Autodesk Inventor part; units mm, degrees
ref_plane "YZ Plane" through (0, 0, 0) normal (1, 0, 0) x (0, 1, 0)
ref_plane "XZ Plane" through (0, 0, 0) normal (0, 1, 0) x (-1, 0, 0)
ref_plane "XY Plane" through (0, 0, 0) normal (0, 0, 1) x (1, 0, 0)
sketch "Sketch1" plane through (0, 0, 0) normal (0, 1, 0) x (-1, 0, 0)
  arc A0 (-2.8605, -1.9692) -> (-1.9692, -2.8605) centre (-2.4696, -2.4696) ccw
  line L0 (-1.3405, -2.2319) -> (-1.9692, -2.8605)
  arc A1 (-1.3405, -2.2319) -> (1.3405, -2.2319) centre (0, 0) ccw
  line L1 (1.9692, -2.8605) -> (1.3405, -2.2319)
  arc A2 (1.9692, -2.8605) -> (2.8605, -1.9692) centre (2.4696, -2.4696) ccw
  line L2 (2.2319, -1.3405) -> (2.8605, -1.9692)
  arc A3 (2.2319, -1.3405) -> (2.2319, 1.3405) centre (0, 0) ccw
  line L3 (2.8605, 1.9692) -> (2.2319, 1.3405)
  arc A4 (2.8605, 1.9692) -> (1.9692, 2.8605) centre (2.4696, 2.4696) ccw
  line L4 (1.3405, 2.2319) -> (1.9692, 2.8605)
  arc A5 (1.3405, 2.2319) -> (-1.3405, 2.2319) centre (0, 0) ccw
  line L5 (-1.9692, 2.8605) -> (-1.3405, 2.2319)
  arc A6 (-1.9692, 2.8605) -> (-2.8605, 1.9692) centre (-2.4696, 2.4696) ccw
  line L6 (-2.2319, 1.3405) -> (-2.8605, 1.9692)
  arc A7 (-2.2319, 1.3405) -> (-2.2319, -1.3405) centre (0, 0) ccw
  line L7 (-2.8605, -1.9692) -> (-2.2319, -1.3405)
  arc A8 (4.5171, -1.6395) -> (5.447, -3.8845) centre (7.6921, -1.6395) ccw
  line L8 (8.7557, -7.1932) -> (5.447, -3.8845)
  arc A9 (8.7557, -7.1932) -> (10.4901, -6.4748) centre (9.4741, -6.4748) ccw
  line L9 (10.4901, 6.4748) -> (10.4901, -6.4748)
  arc A10 (10.4901, 6.4748) -> (8.7557, 7.1933) centre (9.4741, 6.4748) ccw
  line L10 (5.447, 3.8846) -> (8.7557, 7.1933)
  arc A11 (5.447, 3.8846) -> (4.5171, 1.6395) centre (7.6921, 1.6395) ccw
  line L11 (4.5171, -1.6395) -> (4.5171, 1.6395)
  arc A12 (-8.7557, 7.1933) -> (-10.4901, 6.4748) centre (-9.4741, 6.4748) ccw
  line L12 (-10.4901, -6.4747) -> (-10.4901, 6.4748)
  arc A13 (-10.4901, -6.4747) -> (-8.7557, -7.1932) centre (-9.4741, -6.4747) ccw
  line L13 (-5.4471, -3.8845) -> (-8.7557, -7.1932)
  arc A14 (-5.4471, -3.8845) -> (-4.5171, -1.6394) centre (-7.6921, -1.6394) ccw
  line L14 (-4.5171, 1.6395) -> (-4.5171, -1.6394)
  arc A15 (-4.5171, 1.6395) -> (-5.4471, 3.8846) centre (-7.6921, 1.6395) ccw
  line L15 (-8.7557, 7.1933) -> (-5.4471, 3.8846)
  arc A16 (10.5917, -12.6999) -> (12.6999, -10.5917) centre (10.5917, -10.5917) ccw
  line L16 (10.5917, -12.6999) -> (4.356, -12.6999)
  arc A17 (4.356, -10.4901) -> (4.356, -12.6999) centre (4.356, -11.595) ccw
  line L17 (4.356, -10.4901) -> (6.4748, -10.4901)
  arc A18 (6.4748, -10.4901) -> (7.1933, -8.7557) centre (6.4748, -9.4741) ccw
  line L18 (7.1933, -8.7557) -> (3.8846, -5.4471)
  arc A19 (3.8846, -5.4471) -> (1.6395, -4.5171) centre (1.6395, -7.6921) ccw
  line L19 (1.6395, -4.5171) -> (-1.6396, -4.5171)
  arc A20 (-1.6396, -4.5171) -> (-3.8847, -5.4471) centre (-1.6396, -7.6921) ccw
  line L20 (-3.8847, -5.4471) -> (-7.1933, -8.7557)
  arc A21 (-7.1933, -8.7557) -> (-6.4749, -10.4901) centre (-6.4749, -9.4741) ccw
  line L21 (-6.4749, -10.4901) -> (-4.3562, -10.4901)
  arc A22 (-4.3562, -12.6999) -> (-4.3562, -10.4901) centre (-4.3562, -11.595) ccw
  line L22 (-4.3562, -12.6999) -> (-10.5919, -12.6999)
  arc A23 (-12.7001, -10.5917) -> (-10.5919, -12.6999) centre (-10.5919, -10.5917) ccw
  line L23 (-12.7001, -10.5917) -> (-12.7001, 10.5919)
  arc A24 (-10.5919, 12.7001) -> (-12.7001, 10.5919) centre (-10.5919, 10.5919) ccw
  line L24 (-10.5919, 12.7001) -> (-4.3562, 12.7001)
  arc A25 (-4.3562, 10.4903) -> (-4.3562, 12.7001) centre (-4.3562, 11.5952) ccw
  line L25 (-4.3562, 10.4903) -> (-6.475, 10.4903)
  arc A26 (-6.475, 10.4903) -> (-7.1934, 8.7558) centre (-6.475, 9.4743) ccw
  line L26 (-7.1934, 8.7558) -> (-3.8846, 5.4471)
  arc A27 (-3.8846, 5.4471) -> (-1.6396, 4.5172) centre (-1.6396, 7.6922) ccw
  line L27 (-1.6396, 4.5172) -> (1.6395, 4.5172)
  arc A28 (1.6395, 4.5172) -> (3.8845, 5.4471) centre (1.6395, 7.6922) ccw
  line L28 (3.8845, 5.4471) -> (7.1933, 8.7558)
  arc A29 (7.1933, 8.7558) -> (6.4748, 10.4903) centre (6.4748, 9.4743) ccw
  line L29 (6.4748, 10.4903) -> (4.356, 10.4903)
  arc A30 (4.356, 12.7001) -> (4.356, 10.4903) centre (4.356, 11.5952) ccw
  line L30 (4.356, 12.7001) -> (10.5917, 12.7001)
  arc A31 (12.6999, 10.5919) -> (10.5917, 12.7001) centre (10.5917, 10.5919) ccw
  line L31 (12.6999, 10.5919) -> (12.6999, -10.5917)
  point P0 (0, 0)
  dimension "d0" = 2.1082
  dimension "d1" = 1.016
  dimension "d2" = 3.175
  dimension "d3" = 1.1049
  dimension "d4" = 0.635
  dimension "d5" = 2.6035
  dimension "d6" = 2.6035
  dimension "d7" = 2.6035
  dimension "d8" = 2.6035
  dimension "d9" = 90
  dimension "d10" = 90
  dimension "d11" = 45
  dimension "d12" = 45
  dimension "d13" = 45
  dimension "d14" = 90
  dimension "d15" = 90
  dimension "d16" = 45
  dimension "d17" = 45
  dimension "d18" = 45
  dimension "d19" = 45
  dimension "d20" = 45
  dimension "d21" = 45
  dimension "d22" = 2.2099
  dimension "d23" = 8.1829
  dimension "d24" = 17.2171
  dimension "d25" = 23.1901
  dimension "d26" = 25.4
  dimension "d27" = 1.7352
  dimension "d28" = 0.4746
  dimension "d29" = 2.2097
  dimension "d30" = 1.7351
  dimension "d31" = 0.4746
  dimension "d32" = 2.2096
  dimension "d33" = 9.0343
  dimension "d34" = 5.9731
  dimension "d35" = 15.0073
  dimension "d36" = 12.6999
  dimension "d37" = 12.7
  dimension "d38" = 12.6999
  dimension "d39" = 1.1048
  dimension "d40" = 1.1048
  dimension "d41" = 1.1049
  dimension "d42" = 1.1048
  dimension "d43" = 10.4902
  dimension "d44" = 10.4901
  dimension "d45" = 4.5172
  dimension "d46" = 0.6303
  dimension "d47" = 0.6303
  dimension "d48" = 0.6303
  dimension "d49" = 0.6303
  dimension "d50" = 1.1048
  dimension "d51" = 1.1049
  dimension "d52" = 8.3439
  dimension "d53" = 8.3439
  dimension "d54" = 9.8395
  dimension "d55" = 9.8395
  dimension "d56" = 10.2304
  dimension "d57" = 10.2304
  dimension "d58" = 10.4681
  dimension "d59" = 10.4681
  dimension "d60" = 14.6691
  dimension "d61" = 14.6691
  dimension "d62" = 15.1695
  dimension "d63" = 15.1695
extrude "Extrusion1" add sketch "Sketch1" along normal mid plane 25.4
properties part number "1004-S-BLACK-FB" material "6105-T5"
The listing builds one solid part. Answer for the finished solid, in the listing's coordinates (mm). A direction names the side the tool comes from. Coordinates: 2 decimals unless noted, no trailing zeros. Write each loop counter-clockwise with the first axis right and the second up, starting at its lowest first coordinate (ties: lowest second). Pieces come first, ordered by that corner, then holes. Notation, with made-up numbers: M 64,84.25 L 117,84.25 A20 cw 117,112.25 Z; hole C 61,66 d8. An arc over 180 degrees is marked long. Write each question's results on one line, items separated by ' | '.
Item 1: The part is cut by section A-A on x = 10. Determine the outline of the cut face in (y, z), and give its area (3 significant figures).
Answer below:
outline: M -12.7,-12.7 L 12.7,-12.7 L 12.7,-7.34 L -12.7,-7.34 Z; M -12.7,7.34 L 12.7,7.34 L 12.7,12.7 L -12.7,12.7 Z | area: 272 mm2
Item 2: Consider probe 1 along X at (y, z) = (-2.5, 0); probe 2 along X at (y, z) = (11, -3); probe 3 along Z at (x, y) = (-3.5, 9.25). Determine where each line is inside the solid, lowest interval first. Write a range as [from, to].
Answer below:
probe 1: [-12.7, -10.49], [-4.52, -2.6], [2.6, 4.52], [10.49, 12.7] | probe 2: [-12.7, -10.49], [-4.82, -2.82], [-2.12, 2.12], [2.82, 4.82], [10.49, 12.7] | probe 3: [-12.29, -10.9], [-5.12, 5.12], [10.9, 12.29]
Item 3: The part is cut by section B-B on z = -5. Determine the outline of the cut face in (x, y).
Answer below:
outline: M -12.7,-12.7 L -10.49,-12.7 L -10.49,12.7 L -12.7,12.7 Z; M -6.56,-12.7 L -3.32,-12.7 L -3.32,12.7 L -6.56,12.7 Z; M 3.32,-12.7 L 6.56,-12.7 L 6.56,12.7 L 3.32,12.7 Z; M 10.49,-12.7 L 12.7,-12.7 L 12.7,12.7 L 10.49,12.7 Z
Item 4: The part is cut by section D-D on y = 9.25. State how many separate pieces and enclosed holes the cut face has, and give its area (3 significant figures).
Answer below:
separate pieces: 1 | enclosed holes: 3 | area: 310 mm2
Item 5: Given P1, Ø1, axis at x = 0.5, y = -3, coming from the +Z side; P2, Ø1.7, axis at x = -2.47, z = 2.47, coming from the -Y side; P3, Ø3.5, axis at x = 0, y = 3.5, coming from the -Z side, each flat-ended and moving along its own axis, determine where each tip first touches the part or whether it passes through.
Answer below:
P1: z = 4.52 | P2: y = -12.7 | P3: z = -4.52
Item 6: For a pull along X with two mould halves and no side action, classify faces 4 (the face through (2.603, -0.178, -0.02)), 5 (the face through (0, 12.7, 3)), 6 (the face through (-12.099, -0.178, -12.066)) as released by +X, released by -X, zero draft, split by the parting line, or undercut.
Answer below:
face 4: undercut | face 5: zero draft | face 6: released by -X
Item 7: The part is cut by section C-C on z = 3.5. Determine the outline of the cut face in (x, y), and give its area (3 significant figures).
Answer below:
outline: M -12.7,-12.7 L -10.49,-12.7 L -10.49,12.7 L -12.7,12.7 Z; M -5.12,-12.7 L 5.12,-12.7 L 5.12,12.7 L -5.12,12.7 Z; M 10.49,-12.7 L 12.7,-12.7 L 12.7,12.7 L 10.49,12.7 Z | area: 372 mm2
Item 8: Which of the six approach directions +Z, -Z, +X, -X, +Y, -Y give full straight-line access (tool end or side, diameter ignored) to faces 1 (the face through (3.25, -0.18, -11.57)), 2 (the face through (0, 0, -4.517)), 3 (the face through (12.066, -0.178, -12.099))?
Answer below:
face 1: +Y, -Y | face 2: -Z, +Y, -Y | face 3: -Z, +X, +Y, -Y
